The model under review builds one solid part; all positions refer to its coordinate system, in mm. A direction names the side the tool comes from. Coordinates: 2 decimals unless noted, no trailing zeros. Loops run counter-clockwise (first coordinate to the right, second up) from the corner with the lowest first, then second, coordinate; pieces in that order, holes last. Notation, with made-up numbers: (54.25, 69) - (94.25, 69) arc R23 cw to (94.25, 103) - close; hole circle Ø10 at (47.25, -27). An arc over 180 degrees is marked (long way). Answer in a Markdown table with one row per item. Add a question column.
(1) We need section B-B on x = 0. Write out the cut boundary in (y, z) (3 decimals).
(2) Machinability: for faces 1 (the flat face through (2, 0, 1)), 2 (the flat face through (0, 41.275, 0)), which of the approach directions +Z, -Z, +X, -X, +Y, -Y give a long, thin tool a straight path to every point of the face, cutting with its end or side? Answer none if there is none.
(3) We need section C-C on y = 9.5. Write out the cut boundary in (x, z).
(4) For line 1 along Y through (x, z) = (1.75, 0.5); line 2 along Z through (x, y) = (0, 15.5); line 3 along Z through (x, y) = (-0.75, 4.5), list the stretches that pass through material, from the lowest coordinate up.
(5) For P1, Ø2, axis at y = 33, z = -2.5, coming from the +X side; P2, Ø1, axis at y = 19.5, z = 2, coming from the -X side; P3, Ø3, axis at x = -2.5, y = 11.5, coming from the +Z side, all flat-tipped, find the tip position at first contact; note any pin that passes through.
(6) We need section A-A on z = 0. Write out the cut boundary in (x, y) (3 decimals), plus the area to 3 significant figures.
Solid Edge part; units mm, degrees
sketch "Sketch1" plane through (0, 0, 0) normal (0, -1, 0) x (1, 0, 0)
  circle A0 centre (0, 0) radius 1.7526
extrude "Protrusion1" add sketch "Sketch1" against normal blind 41.275
cosmetic_thread "Thread1"
sketch "Sketch2" plane through (0, 0, 0) normal (0, -1, 0) x (1, 0, 0)
  circle A0 centre (0, 0) radius 3.429
extrude "ExtrudedProtrusion_2" add sketch "Sketch2" along normal blind 2.4638
fillet "Round_1" radius 1.524 1 edges at (-3.429, -2.4638, 0)
properties part number "91772A159"
Outcome:
| question | item | result |
|---|---|---|
| 1 | outline | (-2.464, -1.905) arc R1.524 ccw to (-0.94, -3.429) - (0, -3.429) - (0, -1.753) - (41.275, -1.753) - (41.275, 1.753) - (0, 1.753) - (0, 3.429) - (-0.94, 3.429) arc R1.524 ccw to (-2.464, 1.905) - close |
| 2 | face 1 | +Y |
| 2 | face 2 | +Z, -Z, +X, -X, +Y |
| 3 | outline | circle Ø3.51 at (0, 0) |
| 4 | line 1 | -2.46 to 0 |
| 4 | line 2 | -1.75 to 1.75 |
| 4 | line 3 | -1.58 to 1.58 |
| 5 | P1 | x = 0.91 |
| 5 | P2 | x = -0.91 |
| 5 | P3 | z = 1.44 |
| 6 | outline | (-3.429, -0.94) arc R1.524 ccw to (-1.905, -2.464) - (1.905, -2.464) arc R1.524 ccw to (3.429, -0.94) - (3.429, 0) - (1.753, 0) - (1.753, 41.275) - (-1.753, 41.275) - (-1.753, 0) - (-3.429, 0) - close |
| 6 | area | 161 mm² |
